Here's how the part is built. I have some questions about the finished solid (model axes, mm). Face numbers are marked on the shaded views. A direction names the side the tool comes from. Coordinates: 2 decimals unless noted, no trailing zeros. Write each loop counter-clockwise with the first axis right and the second up, starting at its lowest first coordinate (ties: lowest second). Pieces come first, ordered by that corner, then holes. Notation, with made-up numbers: (58, 61) -> (93, 61) arc R21 ccw to (93, 66) -> close; hole circle Ø10 at (-11.75, 25.25). An arc over 180 degrees is marked (long way). Use a Markdown table: item, result. Add a question column.
Autodesk Inventor part; units mm, degrees
ref_plane "YZ Plane" through (0, 0, 0) normal (1, 0, 0) x (0, 1, 0)
ref_plane "XZ Plane" through (0, 0, 0) normal (0, 1, 0) x (-1, 0, 0)
ref_plane "XY Plane" through (0, 0, 0) normal (0, 0, 1) x (1, 0, 0)
sketch "Sketch1" plane through (0, 0, 0) normal (0, 1, 0) x (-1, 0, 0)
  line L0 (0, 0) -> (-85, 0)
  line L1 (-85, 0) -> (-85, 65)
  line L2 (-85, 65) -> (0, 65)
  line L3 (0, 65) -> (0, 0)
  line L4 (-4, 2) -> (-81, 2)
  line L5 (-83, 4) -> (-83, 61)
  line L6 (-81, 63) -> (-4, 63)
  line L7 (-2, 61) -> (-2, 4)
  circle A0 centre (0, 0) radius 2.5
  circle A1 centre (0, 65) radius 2.5
  circle A2 centre (-85, 65) radius 2.5
  circle A3 centre (-85, 0) radius 2.5
  arc A4 (-4, 2) -> (-2, 4) centre (-4, 4) ccw
  arc A5 (-83, 4) -> (-81, 2) centre (-81, 4) ccw
  arc A6 (-81, 63) -> (-83, 61) centre (-81, 61) ccw
  arc A7 (-2, 61) -> (-4, 63) centre (-4, 61) ccw
  point P0 (0, 62.5)
  point P1 (-2.5, 65)
  point P2 (-82.5, 65)
  point P3 (-85, 62.5)
  point P4 (-85, 2.5)
  point P5 (-82.5, 0)
  point P6 (-2.5, 0)
  point P7 (0, 2.5)
  dimension "d0" = 85
  dimension "d1" = 65
  dimension "d14" = 5
  dimension "d15" = 5
  dimension "d16" = 5
  dimension "d17" = 5
  dimension "d18" = 2
extrude "Extrusion1" add sketch "Sketch1" along normal blind 2 contours A3 L1 L0 | A3 L1 A2 L2 A1 L3 A0 L0 | L0 L1 A3 | A0 L3 L0 | L0 L3 A0 | A2 L2 L1 | L1 L2 A2 | A1 L2 L3 | L3 L2 A1 | L4 A5 L5 A6 L6 A7 L7 A4
sketch "Sketch2" plane through (0, 2, 0) normal (0, 1, 0) x (1, 0, 0)
  line L0 (2.5, -65) -> (82.5, -65)
  arc A0 (82.5, -65) -> (85, -62.5) centre (85, -65) ccw
  line L1 (85, -62.5) -> (85, -2.5)
  arc A1 (85, -2.5) -> (82.5, 0) centre (85, 0) ccw
  line L2 (82.5, 0) -> (2.5, 0)
  arc A2 (2.5, 0) -> (0, -2.5) centre (0, 0) ccw
  line L3 (0, -2.5) -> (0, -62.5)
  arc A3 (0, -62.5) -> (2.5, -65) centre (0, -65) ccw
  line L4 (81, -2) -> (4, -2)
  line L5 (2, -4) -> (2, -61)
  line L6 (4, -63) -> (81, -63)
  line L7 (83, -61) -> (83, -4)
  arc A4 (2, -61) -> (4, -63) centre (4, -61) ccw
  arc A5 (4, -2) -> (2, -4) centre (4, -4) ccw
  arc A6 (81, -63) -> (83, -61) centre (81, -61) ccw
  arc A7 (83, -4) -> (81, -2) centre (81, -4) ccw
  dimension "d25" = 2
extrude "Extrusion2" add sketch "Sketch2" along normal blind 55
sketch "Sketch3" plane through (2.5, 0, 65) normal (0, 0, 1) x (1, 0, 0)
  line L0 (11.33, 17.0347) -> (11.33, 40.7227)
  line L1 (17.642, 40.7227) -> (17.642, 17.0347)
  arc A0 (11.33, 17.0347) -> (17.642, 17.0347) centre (14.486, 17.0347) ccw
  arc A1 (17.642, 40.7227) -> (11.33, 40.7227) centre (14.486, 40.7227) ccw
  line L2 (22.6667, 17.0347) -> (22.6667, 40.7227)
  line L3 (28.9787, 40.7227) -> (28.9787, 17.0347)
  arc A2 (22.6667, 17.0347) -> (28.9787, 17.0347) centre (25.8227, 17.0347) ccw
  arc A3 (28.9787, 40.7227) -> (22.6667, 40.7227) centre (25.8227, 40.7227) ccw
  line L4 (32.7043, 17.0347) -> (32.7043, 40.7227)
  line L5 (39.0162, 40.7227) -> (39.0162, 17.0347)
  arc A4 (32.7043, 17.0347) -> (39.0162, 17.0347) centre (35.8602, 17.0347) ccw
  arc A5 (39.0162, 40.7227) -> (32.7043, 40.7227) centre (35.8602, 40.7227) ccw
  line L6 (42.6524, 17.0347) -> (42.6524, 40.7227)
  line L7 (48.9644, 40.7227) -> (48.9644, 17.0347)
  arc A6 (42.6524, 17.0347) -> (48.9644, 17.0347) centre (45.8084, 17.0347) ccw
  arc A7 (48.9644, 40.7227) -> (42.6524, 40.7227) centre (45.8084, 40.7227) ccw
  line L8 (52.6006, 17.0347) -> (52.6006, 40.7227)
  line L9 (58.9125, 40.7227) -> (58.9125, 17.0347)
  arc A8 (52.6006, 17.0347) -> (58.9125, 17.0347) centre (55.7565, 17.0347) ccw
  arc A9 (58.9125, 40.7227) -> (52.6006, 40.7227) centre (55.7565, 40.7227) ccw
  line L10 (62.7271, 17.0347) -> (62.7271, 40.7227)
  line L11 (69.039, 40.7227) -> (69.039, 17.0347)
  arc A10 (62.7271, 17.0347) -> (69.039, 17.0347) centre (65.8831, 17.0347) ccw
  arc A11 (69.039, 40.7227) -> (62.7271, 40.7227) centre (65.8831, 40.7227) ccw
  point P0 (-2.5, 0)
  point P1 (14.486, 28.8787)
  point P2 (25.8227, 28.8787)
  point P3 (35.8602, 28.8787)
  point P4 (45.8084, 28.8787)
  point P5 (55.7565, 28.8787)
  point P6 (65.8831, 28.8787)
extrude "Extrusion3" cut sketch "Sketch3" against normal blind 70
sketch "Sketch4" plane through (0, 0, 2.5) normal (-1, 0, 0) x (0, 0, 1)
  line L0 (0, 0) -> (60, 0)
  line L1 (60, 0) -> (60, 57)
  line L2 (0, 57) -> (60, 57)
  line L3 (0, 0) -> (0, 57)
  line L4 (0, 28.5) -> (10, 28.5)
  line L5 (60, 28.5) -> (49.7848, 28.5)
  point P0 (-2.5, 0)
  dimension "d44" = 10
sketch "Sketch6" plane through (0, 57, 0) normal (0, 1, 0) x (1, 0, 0)
  arc A0 (0, -62.5) -> (2.5, -65) centre (0, -65) ccw
  line L0 (81, -63) -> (4, -63)
  line L1 (2, -61) -> (2, -4)
  circle A1 centre (0, -65) radius 1.5
  line L2 (45.4192, -32.5) -> (-3.1549, -32.5)
  circle A2 centre (0, 0) radius 1.5
  circle A3 centre (85, -65) radius 1.5
  circle A4 centre (85, 0) radius 1.5
  dimension "d45" = 3
  dimension "d48" = 65
  dimension "d51" = 85
extrude "Extrusion4" cut sketch "Sketch6" against normal blind 10
properties part number "Body_Bottom"
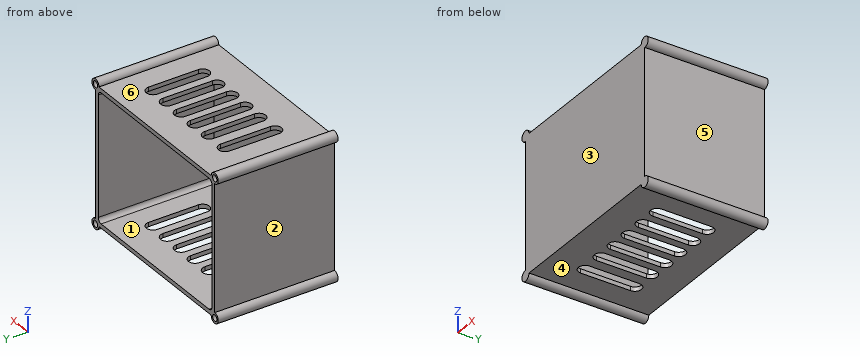
Q1. Suppose I cut it at D-D, the plane y = 23. State how many separate pieces and enclosed holes the cut face has, and give its area (3 significant figures).
Q2. Suppose I cut it at C-C, the plane z = 7. Write out the boundary of the cut face in (x, y).
Q3. Suppose I cut it at A-A, the plane y = 45. Write out the boundary of the cut face in (x, z), and give its area (3 significant figures).
Q4. Thinking about a two-plate mould opening in Z: for the marked faces 4, 5 and 6, which applies, released by +Z, released by -Z, zero draft, split by the parting line, or undercut?
Q5. Which directions (+Z, -Z, +X, -X, +Y, -Y) give clear straight access to the entire face, cutting with the end or side of a thin tool? Please do the marked faces 1, 2 and 3.
Q6. Please list where these lines run through material, in increasing order: line 1 (X direction, y = 42, z = 40); line 2 (Z direction, x = 44, y = 12); line 3 (Y direction, x = 55, z = 30.5).
Q7. Will these pins go through, and if not, where does the flat tip stop? pin 1 (0.6 mm diameter, centred on y = 24, z = 1.5, fed in from +X); pin 2 (1 mm diameter, centred on y = 21, z = 21, fed in from +X); pin 3 (1 mm diameter, centred on y = 32, z = 1.5, fed in from +X).
Q8. Suppose I cut it at B-B, the plane x = 12.5. Write out the boundary of the cut face in (y, z).
Answer key:
| question | item | result |
|---|---|---|
| 1 | separate pieces | 12 |
| 1 | enclosed holes | 0 |
| 1 | area | 495 mm^2 |
| 2 | outline | (0, 0) -> (85, 0) -> (85, 57) -> (83, 57) -> (83, 2) -> (2, 2) -> (2, 57) -> (0, 57) -> close |
| 3 | outline | (0, 2.5) arc R2.5 ccw (long way) to (2.5, 0) -> (82.5, 0) arc R2.5 ccw (long way) to (85, 2.5) -> (85, 62.5) arc R2.5 ccw (long way) to (82.5, 65) -> (2.5, 65) arc R2.5 ccw (long way) to (0, 62.5) -> close; hole (2, 4) arc R2 ccw to (4, 2) -> (81, 2) arc R2 ccw to (83, 4) -> (83, 61) arc R2 ccw to (81, 63) -> (4, 63) arc R2 ccw to (2, 61) -> close |
| 3 | area | 646 mm^2 |
| 4 | face 4 | released by -Z |
| 4 | face 5 | undercut |
| 4 | face 6 | released by +Z |
| 5 | face 1 | +Y |
| 5 | face 2 | -X, +Y, -Y |
| 5 | face 3 | +Z, -Z, +X, -X, -Y |
| 6 | line 1 | x = 0 to 2, 83 to 85 |
| 6 | line 2 | z = 0 to 2, 63 to 65 |
| 6 | line 3 | y = 0 to 2 |
| 7 | pin 1 | stops at x = 87.19 |
| 7 | pin 2 | stops at x = 85 |
| 7 | pin 3 | stops at x = 87.29 |
| 8 | outline | (0, 0) -> (57, 0) -> (57, 2) -> (2, 2) -> (2, 63) -> (57, 63) -> (57, 65) -> (0, 65) -> close |
